Autodesk Inventor part; units mm, degrees
ref_plane "YZ Plane" through (0, 0, 0) normal (1, 0, 0) x (0, 1, 0)
ref_plane "XZ Plane" through (0, 0, 0) normal (0, 1, 0) x (-1, 0, 0)
ref_plane "XY Plane" through (0, 0, 0) normal (0, 0, 1) x (1, 0, 0)
sketch "Sketch1" plane through (0, 0, 0) normal (0, 0, 1) x (1, 0, 0)
  line L0 (100.75, -55.25) -> (169.75, -55.25)
  line L1 (169.75, -55.25) -> (169.75, -124.25)
  line L2 (169.75, -124.25) -> (100.75, -124.25)
  line L3 (100.75, -124.25) -> (100.75, -55.25)
  line L4 (167.75, -122.25) -> (102.75, -122.25)
  line L5 (167.75, -57.25) -> (167.75, -122.25)
  line L6 (102.75, -57.25) -> (167.75, -57.25)
  line L7 (102.75, -122.25) -> (102.75, -57.25)
  point P0 (0, 0)
  dimension "d0" = 69
  dimension "d1" = 69
  dimension "d2" = 2
  dimension "d3" = 2
extrude "Base Shell Extrusion" add sketch "Sketch1" along normal blind 5.25 and the other way blind 5.5 contours L0 L1 L2 L3 | L4 L7 L6 L5
shell "Shell1" thickness 1.75 removed faces 1 at (123.75, -101.25, 5.25)
sketch "USB C Port hole sketch" plane through (100.75, -55.25, 5.25) normal (0, 1, 0) x (1, 0, 0)
  line L0 (19.22, 1.905) -> (22.41, 1.905)
  arc A0 (22.41, 1.905) -> (23.69, 3.185) centre (22.41, 3.185) ccw
  line L1 (23.69, 3.185) -> (23.69, 3.785)
  arc A1 (23.69, 3.785) -> (22.41, 5.065) centre (22.41, 3.785) ccw
  line L2 (22.41, 5.065) -> (19.22, 5.065)
  line L3 (16.03, 5.065) -> (19.22, 5.065)
  arc A2 (16.03, 5.065) -> (14.75, 3.785) centre (16.03, 3.785) ccw
  line L4 (14.75, 3.185) -> (14.75, 3.785)
  arc A3 (14.75, 3.185) -> (16.03, 1.905) centre (16.03, 3.185) ccw
  line L5 (19.22, 1.905) -> (16.03, 1.905)
  arc A4 (22.41, 1.905) -> (23.69, 3.185) centre (22.41, 3.185) ccw
  arc A5 (14.75, 3.185) -> (16.03, 1.905) centre (16.03, 3.185) ccw
  arc A6 (16.03, 5.065) -> (14.75, 3.785) centre (16.03, 3.785) ccw
  arc A7 (23.69, 3.785) -> (22.41, 5.065) centre (22.41, 3.785) ccw
  line L6 (14.75, 3.785) -> (14.75, 3.185)
  line L7 (16.03, 5.065) -> (22.41, 5.065)
  line L8 (23.69, 3.785) -> (23.69, 3.185)
  line L9 (16.03, 1.905) -> (22.41, 1.905)
  line L10 (22.41, 1.405) -> (19.22, 1.405)
  line L11 (19.22, 1.405) -> (16.03, 1.405)
  arc A8 (14.25, 3.185) -> (16.03, 1.405) centre (16.03, 3.185) ccw
  line L12 (14.25, 3.185) -> (14.25, 3.785)
  arc A9 (16.03, 5.565) -> (14.25, 3.785) centre (16.03, 3.785) ccw
  line L13 (16.03, 5.565) -> (19.22, 5.565)
  line L14 (19.22, 5.565) -> (22.41, 5.565)
  arc A10 (24.19, 3.785) -> (22.41, 5.565) centre (22.41, 3.785) ccw
  line L15 (24.19, 3.785) -> (24.19, 3.185)
  arc A11 (22.41, 1.405) -> (24.19, 3.185) centre (22.41, 3.185) ccw
  point P0 (-100.75, 5.25)
  dimension "d24" = 0.5
sketch "Rough encoder hole" plane through (100.75, -124.25, 5.25) normal (0, -1, 0) x (1, 0, 0)
  line L0 (67.25, -7.8767) -> (32.25, -7.8767)
  line L1 (32.25, -7.8767) -> (32.25, 0.1233)
  line L2 (32.25, 0.1233) -> (67.25, 0.1233)
  line L3 (67.25, 0.1233) -> (67.25, -7.8767)
  line L4 (67.25, -9) -> (67.25, 0)
  point P0 (-100.75, -5.25)
  dimension "d13" = 35
  dimension "d14" = 8
  dimension "d17" = 0
extrude "Rough Encoder Hole Extrusion" cut sketch "Rough encoder hole" against normal up to surface (1.75 mm away)
extrude "USB C Hole Extrusion" cut sketch "USB C Port hole sketch" against normal up to surface (1.75 mm away) contours L5 A3 L4 A2 L3 L2 A1 L1 A0 L0 | L10 L11 A8 L12 A9 L13 L14 A10 L15 A11
properties part number "Base REV 1.0"
Build history of the part. All positions in model axes, mm. A direction names the side the tool comes from. Coordinates: 2 decimals unless noted, no trailing zeros. Order: outer loops, then holes, each group sorted by start corner. A loop starts at its lowest first (then second) coordinate and runs counter-clockwise, first axis right, second up.
Item 1: Tool access for faces 5 (the flat face through (133, -56, 5.25)), 6 (the flat face through (169.75, -89, 0)), 7 (the flat face through (151, -123, -2.627)), 8 (the flat face through (121, -122.5, 1)), 9 (the flat face through (120, -56, 3.845)): list every direction of +Z, -Z, +X, -X, +Y, -Y with a clear straight run to the whole face (end or side of a thin tool).
Filled in:
face 5: +Z, +X, -X, +Y, -Y
face 6: +Z, -Z, +X, +Y, -Y
face 7: +Z, -Y
face 8: +Z
face 9: +Y
Item 2: Mould opens along Y. For faces 1 (the flat face through (135, -55.25, 0)), 2 (the flat face through (120, -56, -0.315)), 3 (the flat face through (135, -57, 1)), 4 (the flat face through (102.5, -90, 1)) say: released by +Y, released by -Y, zero draft, split by the parting line, or undercut.
Filled in:
face 1: released by +Y
face 2: zero draft
face 3: undercut
face 4: undercut
Item 3: Drill centre lines: L1, parallel to X at y = -117, z = -0.75; L2, parallel to Y at x = 111, z = 0.25; L3, parallel to Z at x = 137, y = -75. Where is each one in solid material? Low to high.
Filled in:
L1: x = 100.75 to 102.5, 168 to 169.75
L2: y = -124.25 to -122.5, -57 to -55.25
L3: z = -5.5 to -3.75
Item 4: Saw through at B-B on y = -72. List the corners of the cut face in (x, z).
Filled in:
outline: (100.75, -5.5) - (169.75, -5.5) - (169.75, 5.25) - (168, 5.25) - (168, -3.75) - (102.5, -3.75) - (102.5, 5.25) - (100.75, 5.25) - close
Item 5: Saw through at D-D on z = 3. List the corners of the cut face in (x, y).
Filled in:
outline: (100.75, -124.25) - (133, -124.25) - (133, -122.5) - (102.5, -122.5) - (102.5, -57) - (115.27, -57) - (115.27, -55.25) - (100.75, -55.25) - close; (124.67, -57) - (168, -57) - (168, -124.25) - (169.75, -124.25) - (169.75, -55.25) - (124.67, -55.25) - close
Item 6: Saw through at A-A on x = 120.5. List the corners of the cut face in (y, z) (3 decimals), then the cut area to 3 significant figures.
Filled in:
outline: (-124.25, -5.5) - (-55.25, -5.5) - (-55.25, -0.315) - (-57, -0.315) - (-57, -3.75) - (-122.5, -3.75) - (-122.5, 5.25) - (-124.25, 5.25) - close; (-57, 3.845) - (-55.25, 3.845) - (-55.25, 5.25) - (-57, 5.25) - close
area: 145 mm2
Item 7: Drop flat-ended pins along their axis: pin 1 Ø5 at (x, z) = (145, 0.5) entering from -Y; pin 2 Ø1.9 at (x, y) = (147.5, -123) entering from +Z; pin 3 Ø2 at (x, y) = (112, -108.5) entering from +Z. Give the stop position or say it passes through.
Filled in:
pin 1: stops at y = -57
pin 2: stops at z = -2.63
pin 3: stops at z = -3.75
Item 8: Saw through at C-C on x = 113. List the corners of the cut face in (y, z), then the cut area to 3 significant figures.
Filled in:
outline: (-124.25, -5.5) - (-55.25, -5.5) - (-55.25, 5.25) - (-57, 5.25) - (-57, -3.75) - (-122.5, -3.75) - (-122.5, 5.25) - (-124.25, 5.25) - close
area: 152 mm2
